from build123d import *

# Parameters (mm, degrees)
SKETCH_1_R               = 22
EXTRUDE_1_DEPTH          = 2
SKETCH_3_R               = 1.25
CUT_EXTRUDE_1_DEPTH      = 3
SKETCH_4_R               = 3.5
CUT_EXTRUDE_2_DEPTH      = 3
SKETCH_6_R               = 3
EXTRUDE_3_DEPTH          = 9.5
SKETCH_8_R               = 1
CUT_EXTRUDE_4_DEPTH      = 11.5
CUT_EXTRUDE_3_DEPTH      = 6
PATTERN_CIRCULAR_1_COUNT = 4
FILLET_2_R               = 1.5
FILLET_3_R               = 1.5


with BuildPart() as part:
    # 草图1 → 凸台-拉伸1 (new body)
    with BuildSketch(Plane.XY):
        Circle(SKETCH_1_R)
    extrude(amount=EXTRUDE_1_DEPTH)

    # 草图3 → 切除-拉伸1 (cut)
    with BuildSketch(Plane(origin=(0, 0, 0), x_dir=(-1, 0, 0), z_dir=(0, 0, -1))):
        with Locations((6, 0)):
            Circle(SKETCH_3_R)
    cut_extrude_1 = extrude(amount=-CUT_EXTRUDE_1_DEPTH, mode=Mode.SUBTRACT)

    # 草图4 → 切除-拉伸2 (cut)
    with BuildSketch(Plane(origin=(0, 0, 0), x_dir=(-1, 0, 0), z_dir=(0, 0, -1))):
        Circle(SKETCH_4_R)
    extrude(amount=-CUT_EXTRUDE_2_DEPTH, mode=Mode.SUBTRACT)

    # 草图6 → 凸台-拉伸3 (add)
    with BuildSketch(Plane(origin=(0, 0, 0), x_dir=(-1, 0, 0), z_dir=(0, 0, -1))):
        with Locations((0, -19)):
            Circle(SKETCH_6_R)
    extrude_3 = extrude(amount=EXTRUDE_3_DEPTH)

    # 草图8 → 切除-拉伸4 (cut)
    with BuildSketch(Plane(origin=(0, 0, -9.5), x_dir=(-1, 0, 0), z_dir=(0, 0, -1))):
        with Locations((0, -19)):
            Circle(SKETCH_8_R)
    cut_extrude_4 = extrude(amount=-CUT_EXTRUDE_4_DEPTH, mode=Mode.SUBTRACT)

    # 草图7 → 切除-拉伸3 (cut)
    with BuildSketch(Plane(origin=(0, 0, 0), x_dir=(-1, 0, 0), z_dir=(0, 0, -1))):
        Polygon((-2.572740594, 10.290962376), (-10.290962376, 2.572740594), (-30.512752563, 7.628188141), (-7.628188141, 30.512752563), align=None)
    cut_extrude_3 = extrude(amount=-CUT_EXTRUDE_3_DEPTH, mode=Mode.SUBTRACT)

    # 阵列(圆周)1: 切除-拉伸1, 凸台-拉伸3, 切除-拉伸4, 切除-拉伸3 ×4 about axis
    pattern_circular_1_axis = Axis((0, 0, 0), (0, 0, 1))
    for i in range(1, PATTERN_CIRCULAR_1_COUNT):
        add(cut_extrude_1.rotate(pattern_circular_1_axis, i * 360 / PATTERN_CIRCULAR_1_COUNT), mode=Mode.SUBTRACT)
        add(extrude_3.rotate(pattern_circular_1_axis, i * 360 / PATTERN_CIRCULAR_1_COUNT))
        add(cut_extrude_4.rotate(pattern_circular_1_axis, i * 360 / PATTERN_CIRCULAR_1_COUNT), mode=Mode.SUBTRACT)
        add(cut_extrude_3.rotate(pattern_circular_1_axis, i * 360 / PATTERN_CIRCULAR_1_COUNT), mode=Mode.SUBTRACT)

    # 圆角2
    fillet_2_edges = [part.edges().sort_by_distance(p)[0] for p in [
        (-5.335783751, -21.343135003, 1),
        (-21.343135003, -5.335783751, 1),
        (21.343135003, -5.335783751, 1),
        (5.335783751, -21.343135003, 1),
        (5.335783751, 21.343135003, 1),
        (21.343135003, 5.335783751, 1),
        (-21.343135003, 5.335783751, 1),
        (-5.335783751, 21.343135003, 1),
    ]]
    fillet(fillet_2_edges, radius=FILLET_2_R)

    # 圆角3
    fillet_3_edges = [part.edges().sort_by_distance(p)[0] for p in [
        (-10.290962376, -2.572740594, 1),
        (-2.572740594, -10.290962376, 1),
        (2.572740594, -10.290962376, 1),
        (10.290962376, -2.572740594, 1),
        (10.290962376, 2.572740594, 1),
        (2.572740594, 10.290962376, 1),
        (-2.572740594, 10.290962376, 1),
        (-10.290962376, 2.572740594, 1),
    ]]
    fillet(fillet_3_edges, radius=FILLET_3_R)


solid = part.part
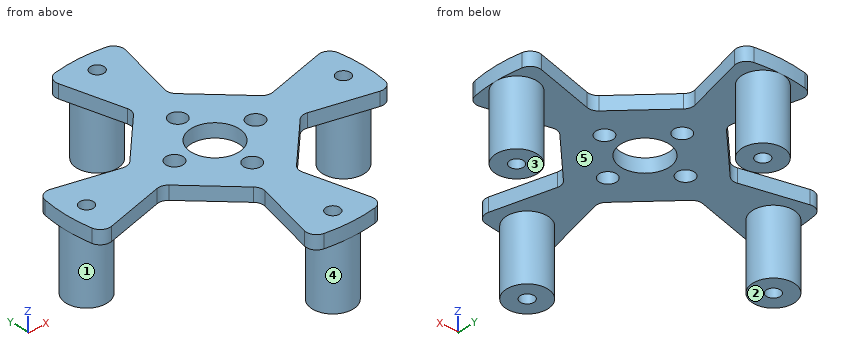
Can you work these out from the model? Positions are in its coordinate system, mm. Face numbers are marked on the shaded views. A direction names the side the tool comes from. Coordinates: 2 decimals unless noted, no trailing zeros. Write each loop counter-clockwise with the first axis right and the second up, starting at its lowest first coordinate (ties: lowest second). Pieces come first, ordered by that corner, then holes.
Q1. For P1, Ø10, axis at x = -5, y = -1, coming from the -Z side; P2, Ø5, axis at y = 1, z = -5.5, coming from the -X side, each with a flat end and sliding along its axis, tell me the tip position at first contact or that it passes through.
Results found:
P1: stops at z = 0
P2: stops at x = -22
Q2. If we mould it in two halves opening along X, with no side actions, what happens to the marked faces 3, 4 and 5? For each: +X half, -X half, draft (parallel to the pull), parting line (faces both ways), or undercut.
Results found:
face 3: draft
face 4: parting line
face 5: undercut
Q3. Which directions (+Z, -Z, +X, -X, +Y, -Y) give clear straight access to the entire face, cutting with the end or side of a thin tool? Please do the marked faces 1 and 2.
Results found:
face 1: -Z
face 2: -Z, +X, -X, +Y, -Y
Q4. Please list where these lines run through material, in increasing order: L1, parallel to Y at x = 0, z = -1.5; L2, parallel to Y at x = 19, z = -0.5; L3, parallel to X at y = -1.5, z = 1.5.
Results found:
L1: y = -22 to -20, -18 to -16, 16 to 18, 20 to 22
L2: y = -3 to -1, 1 to 3
L3: x = -21.95 to -3.16, 3.16 to 21.95
Q5. Imagine slicing it at B-B, the plane y = 19. List the corners of the cut face in (x, z) for me.
Results found:
outline: (-4.75, 0) - (-3, 0) - (-3, -9.5) - (-1, -9.5) - (-1, 2) - (-4.75, 2) - close; (1, -9.5) - (3, -9.5) - (3, 0) - (4.75, 0) - (4.75, 2) - (1, 2) - close
Q6. Imagine slicing it at A-A, the plane z = -6.5. List the corners of the cut face in (x, y) for me, plus the area to 3 significant figures.
Results found:
outline: circle Ø6 at (-19, 0); circle Ø6 at (0, -19); circle Ø6 at (0, 19); circle Ø6 at (19, 0); hole circle Ø2 at (-19, 0); hole circle Ø2 at (0, -19); hole circle Ø2 at (0, 19); hole circle Ø2 at (19, 0)
area: 101 mm2
Q7. Imagine slicing it at D-D, the plane y = 6. List the corners of the cut face in (x, z) for me.
Results found:
outline: (-6.86, 0) - (-1.25, 0) - (-1.25, 2) - (-6.86, 2) - close; (1.25, 0) - (6.86, 0) - (6.86, 2) - (1.25, 2) - close
